Input: part model. Units: mm. Frame: model coordinates. A direction names the side the tool comes from. Give positions to 0.01 mm unless a question says otherwise; leave off trailing zeros. Write each loop counter-clockwise with the first axis right and the second up, starting at its lowest first coordinate (ties: lowest second). Pieces come first, ordered by that corner, then holes. Notation, with made-up numbers: (-39, -17) -> (13, -17) arc R10 ccw to (13, -11) -> close; hole circle Ø11 at (-10.75, 21.5). An arc over 180 degrees is marked (long way). Return JSON: item names as keys, results as strings. Group by question number.
Item 1: Section B-B, the plane x = 64.5. Return loops of the section in (y, z), then the cut area to 3 significant figures.
Item 2: Line query: line 1 (Y direction, x = 72, z = -32); line 2 (Z direction, x = 62, y = -12); line 3 (Y direction, x = 52, z = -103). Output: solid intervals per line, ascending. Write a range as [from, to].
Item 3: Section A-A, the plane z = -32. Return loops of the section in (x, y), then the cut area to 3 significant figures.
Item 4: Mould query, pull axis Y, two halves, no side actions, for faces 1 (the face through (43.724, -29.139, -103.042)), 2 (the face through (56, 0, -36)), 3 (the face through (55.76, -5.74, -86.6)), 4 (the face through (63, -20, -28)). Classes: released by +Y, released by -Y, zero draft, split by the parting line, or undercut.
Item 5: Set-up query: faces 5 (the face through (68, -27, -32)), 6 (the face through (56.131, -41.297, -102.451)), 7 (the face through (62.49, -25.06, -35.49)), 8 (the face through (41.61, -24.49, -102.45)). Return all of +Z, -Z, +X, -X, +Y, -Y with unobstructed straight access to the full face (end or side cutting, diameter ignored); none if empty.
Item 6: Pin query (flat end, axial travel): P1, Ø10, axis at x = 61.5, z = -63.5, coming from the -Y side; P2, Ø3, axis at x = 52.5, z = -89, coming from the +Y side; P3, Ø3, axis at x = 60.5, y = -37, coming from the +Z side. Return the tip coordinate at first contact, or that it passes through.
Item 7: Section D-D, the plane z = -7. Return loops of the section in (x, y), then the cut area to 3 significant figures.
Item 8: Section C-C, the plane y = -41. Return loops of the section in (x, z), then the cut area to 3 significant figures.
from build123d import *

# Parameters (mm, degrees)
BOSS_EXTRUDE1_DEPTH = 37
BOSS_EXTRUDE3_DEPTH = 37
SKETCH5_R           = 11
CUT_EXTRUDE1_DEPTH  = 7
SKETCH6_R           = 10
CUT_EXTRUDE2_DEPTH  = 7
BOSS_EXTRUDE4_START = -37
BOSS_EXTRUDE4_DEPTH = 37
SKETCH8_R           = 9.5
CUT_EXTRUDE3_DEPTH  = 6
SKETCH9_R           = 8
CUT_EXTRUDE4_DEPTH  = 1
CUT_EXTRUDE5_DEPTH  = 7
CUT_EXTRUDE6_DEPTH  = 131.044047905
FILLET2_R           = 10
SKETCH12_R          = 1.5
CUT_EXTRUDE7_DEPTH  = 116.667627277
FILLET5_R           = 15
SKETCH20_R          = 1.5
CUT_EXTRUDE14_DEPTH = 6
SKETCH21_R          = 1
CUT_EXTRUDE15_DEPTH = 6


with BuildPart() as part:
    # Sketch3 → Boss-Extrude1 (new body)
    with BuildSketch(Plane(origin=(0, 0, 0), x_dir=(0, 0, -1), z_dir=(1, 0, 0))):
        with BuildLine():
            Line((0, 0), (73, 0))
            ThreePointArc((73, 0), (96.162469644, -4.825758115), (115.470578051, -18.5))
            Line((115.470578051, -18.5), (109.820510589, -18.5))
            ThreePointArc((109.820510589, -18.5), (107.466378544, -16.429953692), (104.996093512, -14.5))
            ThreePointArc((104.996093512, -14.5), (89.83745824, -6.692105871), (73, -4))
            Line((73, -4), (0, -4))
            Line((0, -4), (0, 0))
        make_face()
    extrude(amount=BOSS_EXTRUDE1_DEPTH)

    # Sketch4 → Boss-Extrude3 (add)
    with BuildSketch(Plane(origin=(37, 0, 0), x_dir=(0, 0, -1), z_dir=(1, 0, 0))):
        Polygon((28, -4), (28, -14.5), (28, -36.5), (28, -47), (36, -47), (36, -35.5), (36, -15.5), (36, -4), align=None)
    extrude(amount=-BOSS_EXTRUDE3_DEPTH)

    # Sketch5 → Cut-Extrude1 (cut)
    with BuildSketch(Plane.XY.offset(-28)):
        with Locations((21.5, -25.5)):
            Circle(SKETCH5_R)
    extrude(amount=-CUT_EXTRUDE1_DEPTH, mode=Mode.SUBTRACT)

    # Sketch6 → Cut-Extrude2 (cut)
    with BuildSketch(Plane.XY.offset(-35)):
        with Locations((21.5, -25.5)):
            Circle(SKETCH6_R)
    extrude(amount=-CUT_EXTRUDE2_DEPTH, mode=Mode.SUBTRACT)

    # Sketch7 → Boss-Extrude4 (add)
    with BuildSketch(Plane(origin=(37, 0, 0), x_dir=(0, 0, -1), z_dir=(1, 0, 0)).offset(BOSS_EXTRUDE4_START)):
        with BuildLine():
            Line((99, -10.671361735), (99, -47))
            Line((99, -47), (106, -47))
            Line((106, -47), (106, -15.256579454))
            ThreePointArc((106, -15.256579454), (102.588951576, -12.82817311), (99, -10.671361735))
        make_face()
    extrude(amount=BOSS_EXTRUDE4_DEPTH)

    # Sketch8 → Cut-Extrude3 (cut)
    with BuildSketch(Plane.XY.offset(-106)):
        with Locations((21.5, -25.5)):
            Circle(SKETCH8_R)
    extrude(amount=CUT_EXTRUDE3_DEPTH, mode=Mode.SUBTRACT)

    # Sketch9 → Cut-Extrude4 (cut)
    with BuildSketch(Plane(origin=(0, 0, -100), x_dir=(-1, 0, 0), z_dir=(0, 0, -1))):
        with Locations((-21.5, -25.5)):
            Circle(SKETCH9_R)
    extrude(amount=-CUT_EXTRUDE4_DEPTH, mode=Mode.SUBTRACT)

    # Sketch10 → Cut-Extrude5 (cut)
    with BuildSketch(Plane(origin=(0, 0, -106), x_dir=(-1, 0, 0), z_dir=(0, 0, -1))):
        Polygon((0, -23.757683827), (-17.471056315, -42.081867062), (-27.318513182, -42.081867062), (-37, -30.228411032), (-37, -47), (0, -47), align=None)
    extrude(amount=-CUT_EXTRUDE5_DEPTH, mode=Mode.SUBTRACT)

    # Sketch11 → Cut-Extrude6 (cut, through all)
    with BuildSketch(Plane(origin=(37, 0, 0), x_dir=(0, 0, -1), z_dir=(1, 0, 0))):
        with BuildLine():
            Line((106, -15.256579454), (106, -10.303039929))
            ThreePointArc((106, -10.303039929), (110.957207174, -14.145120869), (115.470578051, -18.5))
            Line((115.470578051, -18.5), (109.820510589, -18.5))
            ThreePointArc((109.820510589, -18.5), (107.947902211, -16.833944431), (106, -15.256579454))
        make_face()
    extrude(amount=-CUT_EXTRUDE6_DEPTH, mode=Mode.SUBTRACT)

    # Fillet2
    fillet2_edges = [part.edges().sort_by_distance(p)[0] for p in [
        (17.471056315, -42.081867062, -102.5),
        (27.318513182, -42.081867062, -102.5),
    ]]
    fillet(fillet2_edges, radius=FILLET2_R)

    # Sketch12 → Cut-Extrude7 (cut, through all)
    with BuildSketch(Plane.XY.offset(-99)):
        with Locations((21.5, -13.5)):
            Circle(SKETCH12_R)
        with Locations((33.5, -25.5)):
            Circle(SKETCH12_R)
        with Locations((21.5, -37.5)):
            Circle(SKETCH12_R)
        with Locations((9.5, -25.5)):
            Circle(SKETCH12_R)
    extrude(amount=-CUT_EXTRUDE7_DEPTH, mode=Mode.SUBTRACT)

    # Fillet5
    fillet5_edges = [part.edges().sort_by_distance(p)[0] for p in [
        (0, -47, -32),
        (37, -47, -32),
    ]]
    fillet(fillet5_edges, radius=FILLET5_R)

    # Sketch20 → Cut-Extrude14 (cut)
    with BuildSketch(Plane.ZY):
        with Locations((-32, -4)):
            Circle(SKETCH20_R)
        with Locations((-102.5, -16)):
            Circle(SKETCH20_R)
        with Locations((-32, -27)):
            Circle(SKETCH20_R)
    extrude(amount=-CUT_EXTRUDE14_DEPTH, mode=Mode.SUBTRACT)

    # Sketch21 → Cut-Extrude15 (cut)
    with BuildSketch(Plane.XY):
        with Locations((3, -2)):
            Circle(SKETCH21_R)
        with Locations((34, -2)):
            Circle(SKETCH21_R)
    extrude(amount=-CUT_EXTRUDE15_DEPTH, mode=Mode.SUBTRACT)


with BuildPart() as body_2:
    # Mirror1: mirrored copy
    add(part.part.mirror(Plane(origin=(37, -58, -73), x_dir=(0, 0, 1), z_dir=(-1, 0, 0))))


solid = body_2.part
Answer below:
{
 "1": {"outline": "(-45.96, -36) -> (-4, -36) -> (-4, -73) arc R54 cw to (-10.67, -99) -> (-24, -99) -> (-24, -106) -> (-10.3, -106) arc R58 ccw to (0, -73) -> (0, 0) -> (-4, 0) -> (-4, -28) -> (-45.96, -28) -> close; (-33.72, -106) -> (-27, -106) -> (-27, -99) -> (-33.72, -99) -> close", "area": "894 mm2"},
 "2": {"line 1": "y = [-39.48, -28.5], [-25.5, -5.5], [-2.5, 0]", "line 2": "z = [-106, -99], [-36, -28]", "line 3": "y = [-42.08, -38.91], [-36.09, -34.99], [-16.01, -14.91], [-12.09, -8.36]"},
 "3": {"outline": "(37, -32) arc R15 ccw to (52, -47) -> (59, -47) arc R15 ccw to (74, -32) -> (74, -28.5) -> (68, -28.5) -> (68, -25.5) -> (74, -25.5) -> (74, -5.5) -> (68, -5.5) -> (68, -2.5) -> (74, -2.5) -> (74, 0) -> (37, 0) -> close; hole circle Ø22 at (52.5, -25.5)", "area": "1,230 mm2"},
 "4": {"face 1": "undercut", "face 2": "released by +Y", "face 3": "released by -Y", "face 4": "zero draft"},
 "5": {"face 5": "+X", "face 6": "-Z, +X, -Y", "face 7": "+Z", "face 8": "-Z"},
 "6": {"P1": "stops at y = -4", "P2": "stops at y = -1.84", "P3": "stops at z = -28"},
 "7": {"outline": "(37, -4) -> (74, -4) -> (74, 0) -> (37, 0) -> close", "area": "148 mm2"},
 "8": {"outline": "(40, -36) -> (71, -36) -> (71, -28) -> (40, -28) -> close; (46.9, -106) -> (56.77, -106) -> (56.77, -99) -> (46.9, -99) -> close", "area": "317 mm2"}
}
